The model under review builds one solid part; all positions refer to its coordinate system, in mm. A direction names the side the tool comes from. Give positions to 0.01 mm unless a question says otherwise; leave off trailing zeros. Loops run counter-clockwise (first coordinate to the right, second up) from the corner with the lowest first, then second, coordinate; pieces in that order, holes last. Notation, with made-up numbers: M -8.75,89 L 26.25,89 A15 ccw 26.25,115 Z; hole C 82,-27.5 d7. An arc over 180 degrees is marked long. Return JSON: item names as keys, results as strings.
```python
from build123d import *

# Parameters (mm, degrees)
SWEEP_1_PROFILE_R = 0.5


with BuildPart() as part:
    # 扫描1: sweep along a path in 草图1
    with BuildLine(Plane.XY) as sweep_1_path:
        Line((-6.75, 0), (-8.75, 0))
        ThreePointArc((-8.75, 0), (-10.164213562, 0.585786438), (-10.75, 2))
        Line((-10.75, 2), (-10.75, 17))
        ThreePointArc((-10.75, 17), (-10.164213562, 18.414213562), (-8.75, 19))
        Line((-8.75, 19), (8.75, 19))
        ThreePointArc((8.75, 19), (10.164213562, 18.414213562), (10.75, 17))
        Line((10.75, 17), (10.75, 2))
        ThreePointArc((10.75, 2), (10.164213562, 0.585786438), (8.75, 0))
        Line((8.75, 0), (6.75, 0))
    # 扫描1 profile (on start of the path) → 扫描1 (sweep)
    with BuildSketch(Plane(origin=(-6.75, 0, 0), x_dir=(0, -1, 0), z_dir=(-1, 0, 0))):
        Circle(SWEEP_1_PROFILE_R)
    sweep(path=sweep_1_path.line)


solid = part.part
```
1) Consider section C-C on y = 5. Write out the cut boundary in (x, z), then the cut area to 3 significant figures.
From the geometry:
{"outline": "C -10.75,0 d1; C 10.75,0 d1", "area": "1.57 mm²"}
2) Insertion check: pin 1 (4 mm diameter, centred on x = 0, y = 16, fed in from +Z). The pin has a flat end and moves straight along its axis. Give the tip position at first contact, or say it passes through.
From the geometry:
{"pin 1": "through"}
3) Consider section A-A on x = -7.5. Write out the cut boundary in (y, z), then the cut area to 3 significant figures.
From the geometry:
{"outline": "C 0,0 d1; C 19,0 d1", "area": "1.57 mm²"}
4) Wall thickness on L1, parallel to Y at x = 7.75, z = 0.05; L2, parallel to Y at x = 2, z = 0.05; L3, parallel to X at y = 10.25, z = 0.1: over which ranges is each line inside the solid? List them lowest first. Write a range as from..to.
From the geometry:
{"L1": "-0.5..0.5, 18.5..19.5", "L2": "18.5..19.5", "L3": "-11.24..-10.26, 10.26..11.24"}
5) Tool access review of faces 1 (the face through (-10.25, 9.6, 0.02)), 2 (the face through (6.75, 0, 0)): name each direction out of +Z, -Z, +X, -X, +Y, -Y from which nothing blocks a thin tool from reaching the whole face with its end or side.
From the geometry:
{"face 1": "none", "face 2": "+Z, -Z, -Y"}
6) Consider section B-B on z = 0. Write out the cut boundary in (x, y).
From the geometry:
{"outline": "M -11.25,2 A2.5 ccw -8.75,-0.5 L -6.75,-0.5 L -6.75,0.5 L -8.75,0.5 A1.5 cw -10.25,2 L -10.25,17 A1.5 cw -8.75,18.5 L 8.75,18.5 A1.5 cw 10.25,17 L 10.25,2 A1.5 cw 8.75,0.5 L 6.75,0.5 L 6.75,-0.5 L 8.75,-0.5 A2.5 ccw 11.25,2 L 11.25,17 A2.5 ccw 8.75,19.5 L -8.75,19.5 A2.5 ccw -11.25,17 Z"}
7) Consider section D-D on x = 4. Write out the cut boundary in (y, z).
From the geometry:
{"outline": "C 19,0 d1"}
